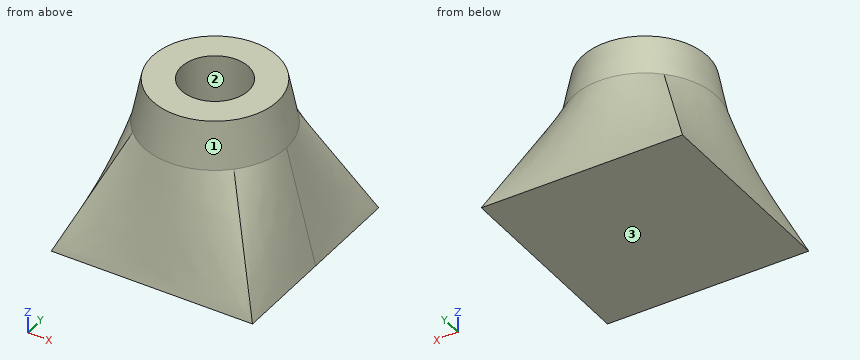
```python
from build123d import *

# Parameters (mm, degrees)
F2_W     = 9
F2_H     = 9
F0_R     = 3.2
F5_R     = 2.8
F7_R     = 1.5
F8_DEPTH = 6.3


with BuildPart() as f3:
    # F2 (on offset) → F3 section 0
    with BuildSketch(Plane.XY.offset(-5)):
        Rectangle(F2_W, F2_H)
    # F0 (on Top) → F3 section 1
    with BuildSketch(Plane.XY):
        Circle(F0_R)
    loft()

    # F0 (on Top) → F6 section 0
    with BuildSketch(Plane.XY):
        Circle(F0_R)
    # F5 (on offset) → F6 section 1
    with BuildSketch(Plane.XY.offset(2)):
        Circle(F5_R)
    loft()

    # F7 (on offset) → F8 (cut)
    with BuildSketch(Plane.XY.offset(2)):
        Circle(F7_R)
    extrude(amount=-F8_DEPTH, mode=Mode.SUBTRACT)


solid = f3.part
```
For this review, take the finished solid that the model builds, in its own axes (mm). Face numbers are marked on the shaded views. Coordinates: 2 decimals unless noted, no trailing zeros. Loops run counter-clockwise (first coordinate to the right, second up) from the corner with the lowest first, then second, coordinate; pieces in that order, holes last. Notation, with made-up numbers: (10, -33.5) - (45, -33.5) arc R15 cw to (45, -19.5) - close; hole circle Ø9 at (27, -23). An arc over 180 degrees is marked (long way). Use one line per item in the form item = value. Start each with the question number.
1) For pin 1 (1 mm diameter, centred on x = 2, z = -1, fed in from +Y); pin 2 (2.5 mm diameter, centred on x = 0, y = 0, fed in from +Z); pin 3 (1 mm diameter, centred on x = -2.5, z = -2.5, fed in from +Y), all flat-tipped, find the tip position at first contact; note any pin that passes through.
2) Draft analysis for pull direction Y (two halves, no side actions). For the marked faces 1, 2 and 3, state which applies: released by +Y, released by -Y, zero draft, split by the parting line, or undercut.
3) Take a section at A-A (z = 0.5). State the section outline as (x, y) points.
4) To check wall thickness, follow probe 1 along Y at (x, z) = (0, -2.75) (3 decimals); probe 2 along Y at (x, z) = (0, -1); probe 3 along X at (y, z) = (-0.5, -2.5). State the ranges of each line that lie inside material, in increasing order. Write a range as from..to.
From the geometry:
q1.pin_1 = 3.34
q1.pin_2 = -4.3
q1.pin_3 = 3.81
q2.face_1 = split by the parting line
q2.face_2 = undercut
q2.face_3 = zero draft
q3.outline = circle Ø6.2 at (0, 0); hole circle Ø3 at (0, 0)
q4.probe_1 = -3.915..-1.5, 1.5..3.915
q4.probe_2 = -3.46..-1.5, 1.5..3.46
q4.probe_3 = -3.84..-1.41, 1.41..3.84
